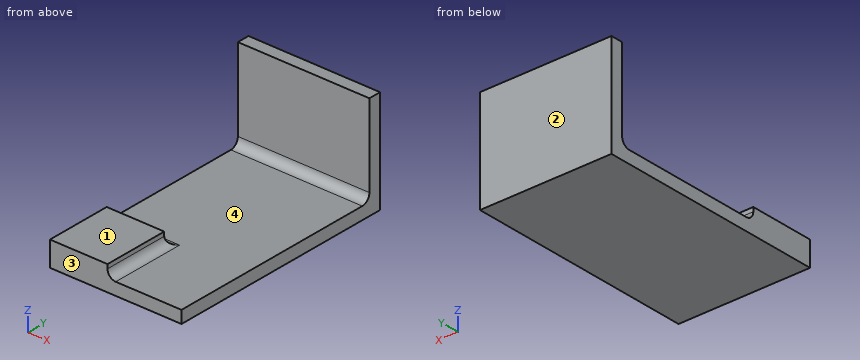
Solid Edge part; units mm, degrees
sketch "Sketch1" plane through (0, 0, 0) normal (0, 0, 1) x (1, 0, 0)
  line L0 (8, -14) -> (8, 14)
  line L1 (8, 14) -> (-8, 14)
  line L2 (-8, 14) -> (-8, -14)
  line L3 (-8, -14) -> (8, -14)
extrude "Protrusion1" add sketch "Sketch1" along normal blind 1.5
sketch "Sketch2" plane through (0, 0, 1.5) normal (0, 0, 1) x (1, 0, 0)
  line L0 (-8, 12.5) -> (8, 12.5)
  line L1 (8, 12.5) -> (8, 14)
  line L2 (8, 14) -> (-8, 14)
  line L3 (-8, 14) -> (-8, 12.5)
extrude "ExtrudedProtrusion_2" add sketch "Sketch2" along normal blind 11
sketch "Sketch3" plane through (0, -1, 1.5) normal (0, 0, 1) x (0, 1, 0)
  line L0 (-5, 1) -> (-5, 8)
  line L1 (-5, 8) -> (-13, 8)
  line L2 (-13, 8) -> (-13, 1)
  line L3 (-13, 1) -> (-5, 1)
extrude "ExtrudedProtrusion_4" add sketch "Sketch3" along normal blind 1.5
fillet "Round1" radius 1 1 edges at (0, 12.5, 1.5)
fillet "Round_3" radius 1 2 edges at (-4.5, -6, 1.5) (-1, -10, 1.5)
Build history of the part. All positions in model axes, mm. Face numbers are marked on the shaded views. Round coordinates to 2 decimals unless told otherwise and drop trailing zeros. Write each loop counter-clockwise with the first axis right and the second up, starting at its lowest first coordinate (ties: lowest second). Pieces come first, ordered by that corner, then holes.
1) Pin check, flat tips, straight feed: pin 1 (5 mm diameter, centred on x = 3, z = 5, fed in from -Y); pin 2 (1.5 mm diameter, centred on x = -3.5, y = 2.5, fed in from +Z); pin 3 (3.5 mm diameter, centred on x = -3, y = -10, fed in from +Z). Stop position of each tip, or through.
2) Band-saw the part on D-D, the plane x = 3.5. List the corners of the cut face in (y, z).
3) Band-saw the part on B-B, the plane y = -7.25. List the corners of the cut face in (x, z).
4) Band-saw the part on A-A, the plane x = -5.5. List the corners of the cut face in (y, z).
5) Drill centre lines: probe 1 along Y at (x, z) = (-2.75, 2.5); probe 2 along Z at (x, y) = (-5, -4); probe 3 along Y at (x, z) = (2.5, 8). Where is each one in solid material? Low to high.
6) Band-saw the part on C-C, the plane z = 4. List the corners of the cut face in (x, y).
7) Mould opens along Y. For the marked faces 1, 2, 3 and 4 say: +Y half, -Y half, draft (parallel to the pull), parting line (faces both ways), or undercut.
Ans:
1. pin 1: stops at y = 12.5
1. pin 2: stops at z = 1.5
1. pin 3: stops at z = 3
2. outline: (-14, 0) - (14, 0) - (14, 12.5) - (12.5, 12.5) - (12.5, 2.5) arc R1 cw to (11.5, 1.5) - (-14, 1.5) - close
3. outline: (-8, 0) - (8, 0) - (8, 1.5) - (0, 1.5) arc R1 cw to (-1, 2.5) - (-1, 3) - (-8, 3) - close
4. outline: (-14, 0) - (14, 0) - (14, 12.5) - (12.5, 12.5) - (12.5, 2.5) arc R1 cw to (11.5, 1.5) - (-5, 1.5) arc R1 cw to (-6, 2.5) - (-6, 3) - (-14, 3) - close
5. probe 1: y = -14 to -6, 12.5 to 14
5. probe 2: z = 0 to 1.5
5. probe 3: y = 12.5 to 14
6. outline: (-8, 12.5) - (8, 12.5) - (8, 14) - (-8, 14) - close
7. face 1: draft
7. face 2: +Y half
7. face 3: -Y half
7. face 4: undercut
